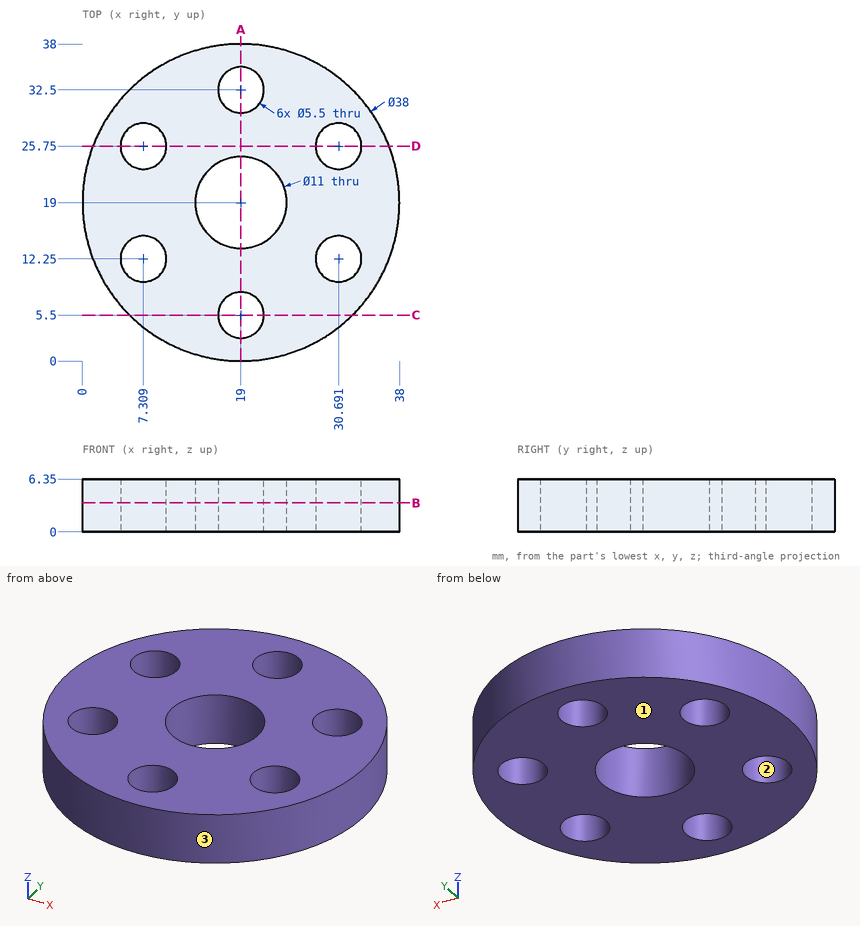
Study the drawing (mm; zero at the part's minimum x, y, z) and answer. Give positions to 0.01 mm unless a question says otherwise; leave off trailing zeros. Write each loop counter-clockwise with the first axis right and the second up, starting at its lowest first coordinate (ties: lowest second). Pieces come first, ordered by that corner, then holes. Notation, with made-up numbers: (86, 3) - (94, 3) arc R7 ccw to (94, 8) - close; hole circle Ø7 at (40.25, 16). An arc over 180 degrees is marked (long way). Write item = value, one per line. Start each with the question number.
Item 1: Find section B-B (z = 3.5). Give the vertices of the cut face in (x, y).
Item 2: Each of these flat-tipped pins is pushed along its axis until it touches: P1, Ø1, axis at y = 20, z = 1.5, coming from the +X side; P2, Ø1, axis at y = 24, z = 3.5, coming from the +X side; P3, Ø1.5, axis at y = 24.5, z = 5, coming from the -X side. Where does it stop, or does it pass through?
Item 3: Find section C-C (y = 5.5). Give the vertices of the cut face in (x, z), then the cut area to 3 significant figures.
Item 4: Find section A-A (x = 19). Give the vertices of the cut face in (y, z), then the cut area to 3 significant figures.
Item 5: Find the intervals of material crossed by probe 1 along Y at (x, z) = (19, 4.25); probe 2 along X at (y, z) = (14.5, 0.75) (1 decimal); probe 3 along X at (y, z) = (25, 2) (1 decimal), in increasing order. Write a range as [from, to].
Item 6: Find section D-D (y = 25.75). Give the vertices of the cut face in (x, z).
Item 7: The mould has two halves that part along X. Classify the marked faces 1, 2 and 3: +X half, -X half, draft (parallel to the pull), parting line (faces both ways), or undercut.
Response:
q1.outline = circle Ø38 at (19, 19); hole circle Ø5.5 at (7.31, 12.25); hole circle Ø5.5 at (7.31, 25.75); hole circle Ø11 at (19, 19); hole circle Ø5.5 at (19, 5.5); hole circle Ø5.5 at (19, 32.5); hole circle Ø5.5 at (30.69, 12.25); hole circle Ø5.5 at (30.69, 25.75)
q2.P1 = 37.99
q2.P2 = 37.46
q2.P3 = 0.6
q3.outline = (5.63, 0) - (16.25, 0) - (16.25, 6.35) - (5.63, 6.35) - close; (21.75, 0) - (32.37, 0) - (32.37, 6.35) - (21.75, 6.35) - close
q3.area = 135 mm²
q4.outline = (0, 0) - (2.75, 0) - (2.75, 6.35) - (0, 6.35) - close; (8.25, 0) - (13.5, 0) - (13.5, 6.35) - (8.25, 6.35) - close; (24.5, 0) - (29.75, 0) - (29.75, 6.35) - (24.5, 6.35) - close; (35.25, 0) - (38, 0) - (38, 6.35) - (35.25, 6.35) - close
q4.area = 102 mm²
q5.probe_1 = [0, 2.75], [8.25, 13.5], [24.5, 29.75], [35.25, 38]
q5.probe_2 = [0.5, 5.7], [8.9, 15.8], [22.2, 29.1], [32.3, 37.5]
q5.probe_3 = [1, 4.7], [10, 28], [33.3, 37]
q6.outline = (1.24, 0) - (4.56, 0) - (4.56, 6.35) - (1.24, 6.35) - close; (10.06, 0) - (27.94, 0) - (27.94, 6.35) - (10.06, 6.35) - close; (33.44, 0) - (36.76, 0) - (36.76, 6.35) - (33.44, 6.35) - close
q7.face_1 = draft
q7.face_2 = undercut
q7.face_3 = parting line
